from build123d import *

# Parameters (mm, degrees)
PAD005_DEPTH  = 3
SKETCH006_W   = 65
SKETCH006_H   = 3
PAD006_DEPTH  = 65
SKETCH007_R   = 2.6
SKETCH007_R_2 = 19.1
POCKET_DEPTH  = 3


with BuildPart() as part:
    # Sketch005 → Pad005 (new body)
    with BuildSketch(Plane.XY):
        Polygon((0, 68.000006), (65, 68.000006), (65, 6.000006), (59, 0), (6, 0), (0, 6.000006), align=None)
        with BuildLine():
            ThreePointArc((50.5, 10), (52.5, 8), (54.5, 10))
            Line((54.5, 10), (54.5, 52))
            ThreePointArc((54.5, 52), (52.5, 54), (50.5, 52))
            Line((50.5, 10), (50.5, 52))
        make_face(mode=Mode.SUBTRACT)
        with BuildLine():
            ThreePointArc((10.5, 10), (12.5, 8), (14.5, 10))
            Line((14.5, 10), (14.5, 52))
            ThreePointArc((14.5, 52), (12.5, 54), (10.5, 52))
            Line((10.5, 10), (10.5, 52))
        make_face(mode=Mode.SUBTRACT)
    extrude(amount=PAD005_DEPTH)

    # Sketch006 (on Face16 of Pad005) → Pad006 (join)
    with BuildSketch(Plane.XY.offset(3)):
        with Locations((32.5, 66.5)):
            Rectangle(SKETCH006_W, SKETCH006_H)
    extrude(amount=PAD006_DEPTH)

    # Sketch007 (on Face21 of Pad006) → Pocket (cut)
    with BuildSketch(Plane.XZ.offset(-65)):
        with Locations((9, 59)):
            Circle(SKETCH007_R)
        with Locations((32.5, 35.5)):
            Circle(SKETCH007_R_2)
        with Locations((56, 12)):
            Circle(SKETCH007_R)
        with Locations((56, 59)):
            Circle(SKETCH007_R)
        with Locations((56, 12)):
            Circle(SKETCH007_R)
        with Locations((9, 12)):
            Circle(SKETCH007_R)
        with Locations((9, 12)):
            Circle(SKETCH007_R)
        Polygon((0, 68), (6, 68), (0, 62), align=None)
        Polygon((65, 68), (59, 68), (65, 62), align=None)
    extrude(amount=-POCKET_DEPTH, mode=Mode.SUBTRACT)


with BuildPart() as part_1:
    # Body005 placement: moved
    add(part.part.moved(Location((12, 0, 0))))


solid = part_1.part
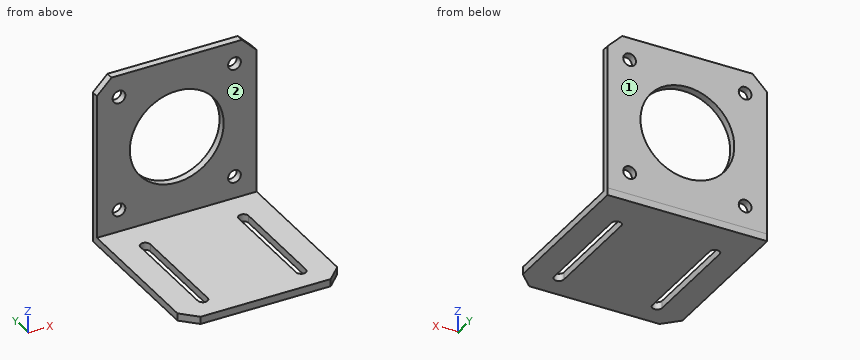
Check sheet for the modelled part. Datum: model origin and axes. Units: mm. Face numbers are marked on the shaded views. A direction names the side the tool comes from. Give positions to 0.01 mm unless a question says otherwise; leave off trailing zeros. Loops run counter-clockwise (first coordinate to the right, second up) from the corner with the lowest first, then second, coordinate; pieces in that order, holes last. Notation, with made-up numbers: M 2,39.5 L 6,39.5 A17 ccw 6,61.5 Z; hole C 3,27.25 d7. An arc over 180 degrees is marked long. Return JSON: item names as keys, results as strings. Group by question number.
1. Cross-section at A-A on z = 59. Record the boundary of the cut face in (x, y).
2. Go/stop test with flat-tipped pins: pin 1 (1.5 mm diameter, centred on x = 67.5, z = 43, fed in from -Y); pin 2 (12 mm diameter, centred on x = 49, z = 28, fed in from -Y); pin 3 (1 mm diameter, centred on x = 29, y = 26, fed in from +Z); pin 4 (8.5 mm diameter, centred on x = 68, z = 12, fed in from +Y). Record where each tip stops, or that it passes through.
3. Cross-section at D-D on z = 25.5. Record the boundary of the cut face in (x, y).
4. Thickness scan on L1, parallel to Z at x = 68, y = 66; L2, parallel to Z at x = 44.5, y = 67.25; L3, parallel to X at y = 67, z = 35. Record the ranges inside material, lowest first.
5. Cross-section at C-C on y = 32.5. Record the boundary of the cut face in (x, z), plus the area to 3 significant figures.
6. Tool access check on the marked faces 1 and 2. Record the directions out of +Z, -Z, +X, -X, +Y, -Y that give a thin tool (end or side, any length) a straight path to the whole face; none if there is none.
7. Cross-section at B-B on x = 21. State how many separate pieces and enclosed holes the cut face has, plus the area to 3 significant figures.
Return value:
{
 "1": {"outline": "M 12,65 L 18.4,65 L 18.4,68 L 12,68 Z; M 23.6,65 L 65.4,65 L 65.4,68 L 23.6,68 Z; M 70.6,65 L 77,65 L 77,68 L 70.6,68 Z"},
 "2": {"pin 1": "y = 65", "pin 2": "through", "pin 3": "z = 3", "pin 4": "y = 68"},
 "3": {"outline": "M 12,65 L 28.23,65 L 28.23,68 L 12,68 Z; M 60.77,65 L 77,65 L 77,68 L 60.77,68 Z"},
 "4": {"L1": "0 to 9.4, 14.6 to 56.4, 61.6 to 68", "L2": "0 to 16.4, 54.6 to 68", "L3": "12 to 25.41, 63.59 to 77"},
 "5": {"outline": "M 12,0 L 22.5,0 L 22.5,3 L 12,3 Z; M 26.5,0 L 62.5,0 L 62.5,3 L 26.5,3 Z; M 66.5,0 L 77,0 L 77,3 L 66.5,3 Z", "area": "171 mm^2"},
 "6": {"face 1": "+Z, -Z, +X, -X, +Y", "face 2": "+Z, +X, -X, -Y"},
 "7": {"separate pieces": "3", "enclosed holes": "0", "area": "368 mm^2"}
}
